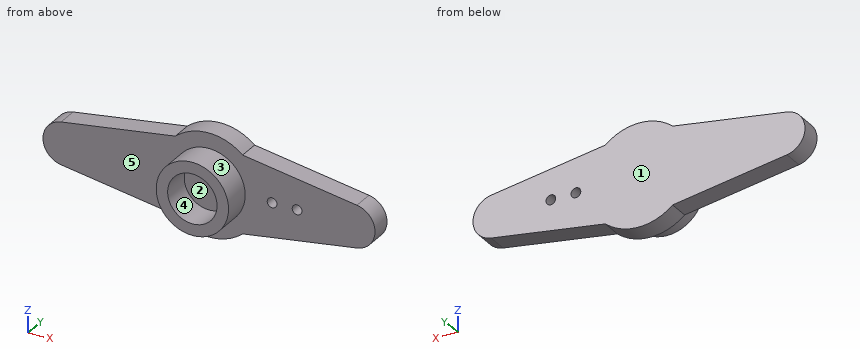
```python
from build123d import *

# Parameters (mm, degrees)
BOSS_EXTRUDE1_DEPTH = 2.413
SKETCH2_R           = 4.22275
SKETCH2_R_2         = 2.8829
BOSS_EXTRUDE2_DEPTH = 3.3401
CUT_EXTRUDE1_REACH  = 7.753
SKETCH3_R           = 0.5715


with BuildPart() as part:
    # Sketch1 → Boss-Extrude1 (new body)
    with BuildSketch(Plane(origin=(0, 0, 0), x_dir=(1, 0, 0), z_dir=(0, 1, 0))):
        with BuildLine():
            Line((3.926025834, 4.5466), (17.264827457, 2.47015))
            ThreePointArc((17.264827457, 2.47015), (19.3802, 0), (17.264827457, -2.47015))
            Line((17.264827457, -2.47015), (3.926025834, -4.5466))
            ThreePointArc((3.926025834, -4.5466), (0, -6.0071), (-3.926025834, -4.5466))
            Line((-3.926025834, -4.5466), (-17.264827457, -2.47015))
            ThreePointArc((-17.264827457, -2.47015), (-19.3802, 0), (-17.264827457, 2.47015))
            Line((-17.264827457, 2.47015), (-3.926025834, 4.5466))
            ThreePointArc((-3.926025834, 4.5466), (0, 6.0071), (3.926025834, 4.5466))
        make_face()
    extrude(amount=BOSS_EXTRUDE1_DEPTH)

    # Sketch2 → Boss-Extrude2 (add)
    with BuildSketch(Plane.XZ):
        Circle(SKETCH2_R)
        Circle(SKETCH2_R_2, mode=Mode.SUBTRACT)
    extrude(amount=BOSS_EXTRUDE2_DEPTH)

    # Sketch3 → Cut-Extrude1 (cut, up to next)
    with BuildSketch(Plane(origin=(0, 2.413, 0), x_dir=(1, 0, 0), z_dir=(0, 1, 0)), mode=Mode.PRIVATE) as cut_extrude1_sk1:
        with Locations((7.366, 0)):
            Circle(SKETCH3_R)
    cut_extrude1_tool1 = extrude(cut_extrude1_sk1.sketch, amount=-CUT_EXTRUDE1_REACH, mode=Mode.PRIVATE) & part.part
    add(cut_extrude1_tool1.solids().sort_by_distance((7.366, 2.413, 0))[0], mode=Mode.SUBTRACT)
    # Sketch3 → Cut-Extrude1 (cut, up to next)
    with BuildSketch(Plane(origin=(0, 2.413, 0), x_dir=(1, 0, 0), z_dir=(0, 1, 0)), mode=Mode.PRIVATE) as cut_extrude1_sk2:
        with Locations((10.287, 0)):
            Circle(SKETCH3_R)
    cut_extrude1_tool2 = extrude(cut_extrude1_sk2.sketch, amount=-CUT_EXTRUDE1_REACH, mode=Mode.PRIVATE) & part.part
    add(cut_extrude1_tool2.solids().sort_by_distance((10.287, 2.413, 0))[0], mode=Mode.SUBTRACT)


solid = part.part
```
For this review, take the finished solid that the model builds, in its own axes (mm). Face numbers are marked on the shaded views. A direction names the side the tool comes from. Round coordinates to 2 decimals unless told otherwise and drop trailing zeros. Write each loop counter-clockwise with the first axis right and the second up, starting at its lowest first coordinate (ties: lowest second). Pieces come first, ordered by that corner, then holes. Notation, with made-up numbers: (-16, 55) -> (5, 55) arc R7 ccw to (5, 62) -> close; hole circle Ø3 at (-1.5, 86). An arc over 180 degrees is marked (long way). Use one line per item in the form item = value.
1) Clearance check with flat-ended pins moving along their axes: pin 1 (1.7 mm diameter, centred on x = 0.5, z = -0.5, fed in from -Y); pin 2 (1 mm diameter, centred on y = -2, z = -1, fed in from +X); pin 3 (0.7 mm diameter, centred on x = 10.287, z = 0, fed in from +Y); pin 4 (1 mm diameter, centred on x = -12.5, y = 1.5, fed in from -Z). State where each tip first meets the part, or that it passes through.
Found:
pin_1 = 0
pin_2 = 4.19
pin_3 = through
pin_4 = -3.29
2) Take a section at A-A, the plane z = 0. Write out the cut boundary in (x, y).
Found:
outline = (-19.38, 0) -> (-4.22, 0) -> (-4.22, -3.34) -> (-2.88, -3.34) -> (-2.88, 0) -> (2.88, 0) -> (2.88, -3.34) -> (4.22, -3.34) -> (4.22, 0) -> (6.79, 0) -> (6.79, 2.41) -> (-19.38, 2.41) -> close; (7.94, 0) -> (9.72, 0) -> (9.72, 2.41) -> (7.94, 2.41) -> close; (10.86, 0) -> (19.38, 0) -> (19.38, 2.41) -> (10.86, 2.41) -> close
3) Take a section at B-B, the plane y = 0.35. Write out the cut boundary in (x, z), and give its area (3 significant figures).
Found:
outline = (-17.26, -2.47) -> (-3.93, -4.55) arc R6.01 ccw to (3.93, -4.55) -> (17.26, -2.47) arc R2.5 ccw to (17.26, 2.47) -> (3.93, 4.55) arc R6.01 ccw to (-3.93, 4.55) -> (-17.26, 2.47) arc R2.5 ccw to start; hole circle Ø1.14 at (7.37, 0); hole circle Ø1.14 at (10.29, 0)
area = 288 mm2
4) To check wall thickness, follow L1, parallel to X at y = 1, z = 0; L2, parallel to Z at x = 0, y = -1.8; L3, parallel to X at y = 1.7, z = -0.5. State the ranges of each line that lie inside material, in increasing order. Write a range as from..to.
Found:
L1 = -19.38..6.79, 7.94..9.72, 10.86..19.38
L2 = -4.22..-2.88, 2.88..4.22
L3 = -19.33..7.09, 7.64..10.01, 10.56..19.33
5) Tool access review of the marked faces 1 and 2: name each direction out of +Z, -Z, +X, -X, +Y, -Y from which nothing blocks a thin tool from reaching the whole face with its end or side.
Found:
face_1 = +Z, -Z, +X, -X, +Y
face_2 = -Y
6) Take a section at C-C, the plane x = 0. Write out the cut boundary in (y, z), and give its area (3 significant figures).
Found:
outline = (-3.34, -4.22) -> (0, -4.22) -> (0, -6.01) -> (2.41, -6.01) -> (2.41, 6.01) -> (0, 6.01) -> (0, 4.22) -> (-3.34, 4.22) -> (-3.34, 2.88) -> (0, 2.88) -> (0, -2.88) -> (-3.34, -2.88) -> close
area = 37.9 mm2
7) Mouldability with a two-part tool opening along X and no side actions: class the marked faces 3, 4 and 5 as +X half, -X half, draft (parallel to the pull), parting line (faces both ways), or undercut.
Found:
face_3 = parting line
face_4 = undercut
face_5 = draft
8) Take a section at D-D, the plane y = -2.05. Write out the cut boundary in (x, z), and give its area (3 significant figures).
Found:
outline = circle Ø8.45 at (0, 0); hole circle Ø5.77 at (0, 0)
area = 29.9 mm2
